Drawing for the job (mm, zero at the part's lowest x, y, z). A direction names the side the tool comes from. Give positions to 0.01 mm unless a question says otherwise; leave off trailing zeros. Order: outer loops, then holes, each group sorted by start corner. A loop starts at its lowest first (then second) coordinate and runs counter-clockwise, first axis right, second up. Notation, with made-up numbers: (46.5, -5) -> (88.5, -5) arc R20 cw to (88.5, 5) -> close; hole circle Ø3 at (-38.75, 80). An arc over 180 degrees is marked (long way). Use a Markdown table: item, result. Add a question column.
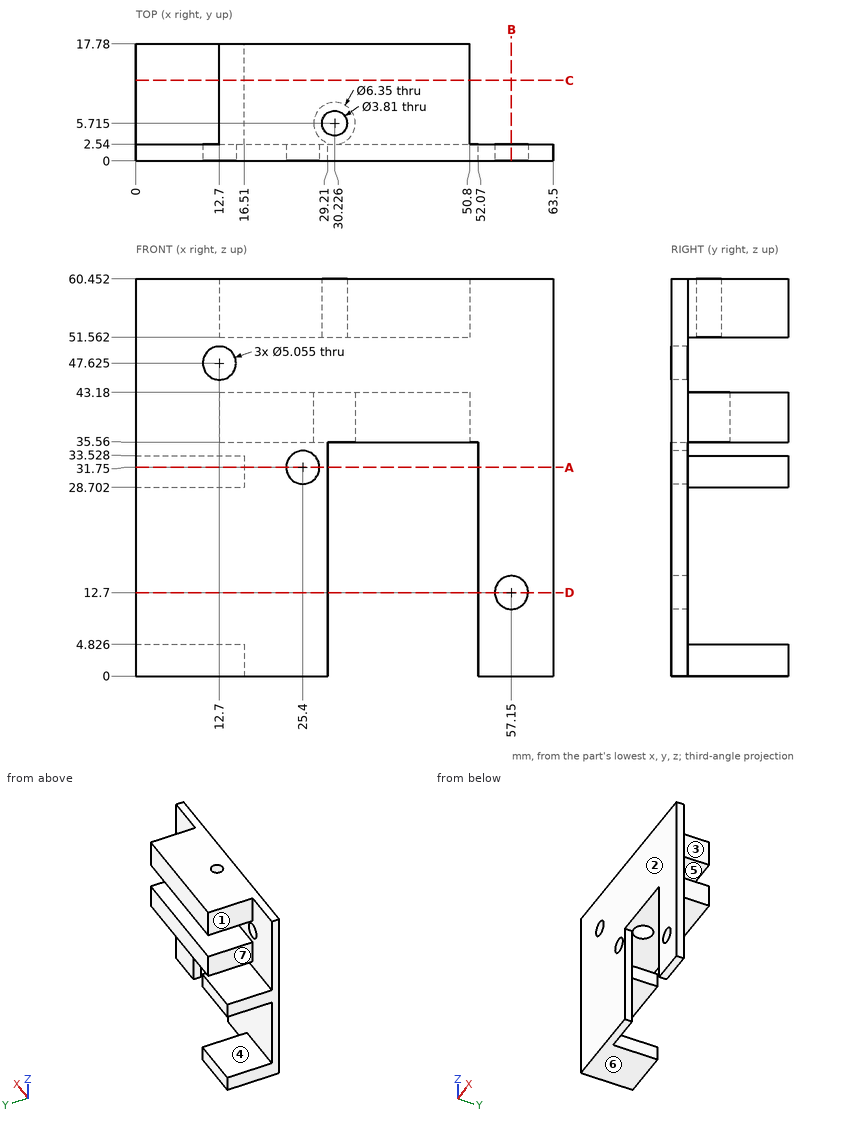
(1) Mould opens along Z. For the marked faces 5, 6 and 7 say: released by +Z, released by -Z, zero draft, split by the parting line, or undercut.
(2) Band-saw the part on B-B on x = 57.15. Give the cut face in (y, z), plus the area to 3 significant figures.
(3) Band-saw the part on A-A on z = 31.75. Give the cut face in (x, y).
(4) Tool access for the marked faces 1, 2, 3 and 4: list every direction of +Z, -Z, +X, -X, +Y, -Y with a clear straight run to the whole face (end or side of a thin tool).
(5) Pin check, flat tips, straight feed: pin 1 Ø6 at (y, z) = (13, 41) entering from +X; pin 2 Ø1.4 at (y, z) = (9, 3.5) entering from +X; pin 3 Ø4 at (x, z) = (52, 22) entering from +Y. Stop position of each tip, or through.
(6) Band-saw the part on C-C on y = 12.25. Give the cut face in (x, z).
(7) Band-saw the part on D-D on z = 12.7. Give the cut face in (x, y).
(8) Wall check: probe 1 along X at (y, z) = (1.75, 31.75); probe 2 along Z at (x, y) = (42, 7); probe 3 along X at (y, z) = (1.5, 47.5) (1 decimal). Give the ranges that are in metal, low to high.
Response:
| question | item | result |
|---|---|---|
| 1 | face 5 | undercut |
| 1 | face 6 | released by -Z |
| 1 | face 7 | zero draft |
| 2 | outline | (0, 0) -> (2.54, 0) -> (2.54, 10.17) -> (0, 10.17) -> close; (0, 15.23) -> (2.54, 15.23) -> (2.54, 60.45) -> (0, 60.45) -> close |
| 2 | area | 141 mm² |
| 3 | outline | (0, 0) -> (22.87, 0) -> (22.87, 2.54) -> (16.51, 2.54) -> (16.51, 17.78) -> (0, 17.78) -> close; (27.93, 0) -> (29.21, 0) -> (29.21, 2.54) -> (27.93, 2.54) -> close; (52.07, 0) -> (63.5, 0) -> (63.5, 2.54) -> (52.07, 2.54) -> close |
| 4 | face 1 | +Z, -X, +Y |
| 4 | face 2 | +Z, -Z, +X, -X, -Y |
| 4 | face 3 | +Z, -Z, +X, +Y |
| 4 | face 4 | +X, -X, +Y |
| 5 | pin 1 | stops at x = 50.8 |
| 5 | pin 2 | stops at x = 16.51 |
| 5 | pin 3 | stops at y = 2.54 |
| 6 | outline | (0, 0) -> (16.51, 0) -> (16.51, 4.83) -> (0, 4.83) -> close; (0, 28.7) -> (16.51, 28.7) -> (16.51, 33.53) -> (0, 33.53) -> close; (12.7, 35.56) -> (50.8, 35.56) -> (50.8, 43.18) -> (12.7, 43.18) -> close; (12.7, 51.56) -> (50.8, 51.56) -> (50.8, 60.45) -> (12.7, 60.45) -> close |
| 7 | outline | (0, 0) -> (29.21, 0) -> (29.21, 2.54) -> (0, 2.54) -> close; (52.07, 0) -> (54.62, 0) -> (54.62, 2.54) -> (52.07, 2.54) -> close; (59.68, 0) -> (63.5, 0) -> (63.5, 2.54) -> (59.68, 2.54) -> close |
| 8 | probe 1 | x = 0 to 22.87, 27.93 to 29.21, 52.07 to 63.5 |
| 8 | probe 2 | z = 35.56 to 43.18, 51.56 to 60.45 |
| 8 | probe 3 | x = 0 to 10.2, 15.2 to 63.5 |
